Geometry check sheet. Reference: the model listing, model coordinates, mm. A direction names the side the tool comes from. Give positions to 0.01 mm unless a question says otherwise; leave off trailing zeros. Order: outer loops, then holes, each group sorted by start corner. A loop starts at its lowest first (then second) coordinate and runs counter-clockwise, first axis right, second up. Notation, with made-up numbers: M 33.25,7.25 L 51.25,7.25 A21 cw 51.25,41.25 Z; hole C -13.5,89.25 d2. An arc over 180 degrees is marked long. Answer as CSV lines item,"result". Start each with the question number.
Q1. Set-up check for faces 5 (the flat face through (-1, 16, -41)), 6 (the flat face through (-1, 10, -17)), 7 (the flat face through (-1, 29, -41)), 8 (the flat face through (1, 6.9, -41)): record each of +Z, -Z, +X, -X, +Y, -Y from which the full face is reachable in a straight line by a thin tool's end or side.
Q2. Mould release check, pull along Z, two halves, no side actions. Record for faces 1 (the flat face through (-1, 22, -53.532)), 2 (the flat face through (-1, 22, 70.568)), 3 (the flat face through (-3.591, 22, 8)), 4 (the flat face through (-1, 8, -43.793)): +Z half, -Z half, draft (parallel to the pull), parting line (faces both ways), or undercut.
Q3. Section check B-B, the plane z = -14. Record the boundary of the cut face in (x, y).
Q4. Go/stop test with flat-tipped pins: pin 1 (2 mm diameter, centred on x = -0.59, z = -41.19, fed in from -Y); pin 2 (1.4 mm diameter, centred on x = -0.5, z = 58, fed in from +Y). Record where each tip stops, or that it passes through.
Q5. Section check A-A, the plane y = 31.5. Record the boundary of the cut face in (x, z), then the cut area to 3 significant figures.
Q6. Thickness scan on line 1 (Z direction, x = -2.4, y = 4.5); line 2 (Y direction, x = 1.45, z = -43); line 3 (Z direction, x = 0.25, y = 7.5). Record the ranges inside material, lowest first.
Autodesk Inventor part; units mm, degrees
ref_plane "YZ Plane" through (0, 0, 0) normal (1, 0, 0) x (0, 1, 0)
ref_plane "XZ Plane" through (0, 0, 0) normal (0, 1, 0) x (-1, 0, 0)
ref_plane "XY Plane" through (0, 0, 0) normal (0, 0, 1) x (1, 0, 0)
sketch "스케치1" plane through (0, 0, 0) normal (0, 1, 0) x (-1, 0, 0)
  line L0 (3.5912, -53.5318) -> (3.5912, 70.5682)
  line L1 (3.5912, -53.5318) -> (-2.4088, -53.5318)
  line L2 (-2.4088, -53.5318) -> (-2.4088, 70.5682)
  line L3 (-2.4088, 70.5682) -> (3.5912, 70.5682)
  line L4 (3.5912, 70.5682) -> (3.5912, -53.5318)
  point P0 (0, 0)
  dimension "d0" = 6
extrude "돌출1" add sketch "스케치1" along normal blind 45
sketch "스케치2" plane through (0, 45, 0) normal (0, 1, 0) x (1, 0, 0)
  line L0 (2.4088, -70.5682) -> (2.4088, 53.5318)
  line L1 (2.4088, -70.5682) -> (-3.5912, -70.5682)
  line L2 (-3.5912, -70.5682) -> (-3.5912, 53.5318)
  line L3 (-3.5912, 53.5318) -> (2.4088, 53.5318)
  line L4 (2.4088, 53.5318) -> (2.4088, -70.5682)
  circle A0 centre (-0.5912, -58.2682) radius 1.35
  circle A1 centre (-0.5912, 41.1925) radius 1.35
  line L5 (2.4088, -70.5682) -> (2.4088, 53.5318)
  line L6 (2.4088, 53.5318) -> (-3.5912, 53.5318)
  line L7 (-3.5912, 53.5318) -> (-3.5912, -70.5682)
  line L8 (-3.5912, -70.5682) -> (2.4088, -70.5682)
  point P0 (0, 0)
  dimension "d3" = 6
  dimension "d4" = 2.7
  dimension "d5" = 2.7
extrude "돌출2" cut sketch "스케치2" against normal blind 16 contours A0 | A1
sketch "스케치3" plane through (2.4088, 0, 70.5682) normal (1, 0, 0) x (0, 0, -1)
  line L0 (0, 0) -> (124.1, 0)
  line L1 (124.1, 0) -> (124.1, 45)
  line L2 (0, 45) -> (124.1, 45)
  line L3 (0, 0) -> (0, 45)
  line L4 (62.05, 0) -> (77.05, 0)
  line L5 (77.05, 0) -> (47.05, 0)
  line L6 (77.05, 0) -> (97.05, 0)
  line L7 (97.05, 0) -> (97.05, 10)
  line L8 (97.05, 10) -> (77.05, 10)
  line L9 (77.05, 10) -> (77.05, 0)
  line L10 (47.05, 0) -> (27.05, 0)
  line L11 (27.05, 0) -> (27.05, 10)
  line L12 (27.05, 10) -> (47.05, 10)
  line L13 (47.05, 10) -> (47.05, 0)
  point P0 (70.5682, 0)
  dimension "d8" = 15
  dimension "d9" = 30
  dimension "d10" = 20
  dimension "d11" = 10
  dimension "d12" = 20
  dimension "d13" = 10
extrude "돌출3" cut sketch "스케치3" against normal blind 16 contours L11 L12 L13 L0 | L9 L8 L7 L0
sketch "스케치4" plane through (0, 0, 0) normal (0, -1, 0) x (1, 0, 0)
  circle A0 centre (-0.5912, 58.2682) radius 1.35
  circle A1 centre (-0.5912, -41.1925) radius 1.35
  point P0 (0, 0)
extrude "돌출4" cut sketch "스케치4" against normal blind 16
sketch "스케치5" plane through (2.4088, 0, -53.5318) normal (1, 0, 0) x (0, 0, -1)
  line L0 (-97.05, 0) -> (-124.1, 0)
  line L1 (-124.1, 0) -> (-97.05, 0)
  line L2 (-27.05, 0) -> (0, 0)
  line L3 (0, 45) -> (-124.1, 45)
  line L4 (-124.1, 45) -> (0, 45)
  line L5 (-113.15, 45) -> (-110.45, 45)
  line L6 (-13.6892, 45) -> (-10.9892, 45)
  line L7 (-124.1, 45) -> (0, 45)
  line L8 (0, 45) -> (-124.1, 45)
  line L9 (-47.05, 10) -> (-47.05, 0)
  line L10 (-47.05, 0) -> (-77.05, 0)
  line L11 (-77.05, 0) -> (-77.05, 10)
  line L12 (-77.05, 10) -> (-97.05, 10)
  line L13 (-97.05, 10) -> (-97.05, 0)
  line L14 (-97.05, 0) -> (-124.1, 0)
  line L15 (-124.1, 0) -> (-124.1, 45)
  line L16 (0, 45) -> (-124.1, 45)
  line L17 (0, 0) -> (0, 45)
  line L18 (0, 0) -> (-27.05, 0)
  line L19 (-27.05, 0) -> (-27.05, 10)
  line L20 (-27.05, 10) -> (-47.05, 10)
  line L21 (-47.05, 0) -> (-47.05, 10)
  line L22 (-47.05, 10) -> (-27.05, 10)
  line L23 (-27.05, 10) -> (-27.05, 0)
  line L24 (-27.05, 0) -> (0, 0)
  line L25 (0, 0) -> (0, 45)
  line L26 (-124.1, 45) -> (0, 45)
  line L27 (-124.1, 0) -> (-124.1, 45)
  line L28 (-124.1, 0) -> (-97.05, 0)
  line L29 (-97.05, 0) -> (-97.05, 10)
  line L30 (-97.05, 10) -> (-77.05, 10)
  line L31 (-77.05, 10) -> (-77.05, 0)
  line L32 (-77.05, 0) -> (-47.05, 0)
  line L33 (-97.05, 10) -> (-77.05, 10)
  line L34 (-77.05, 10) -> (-97.05, 10)
  line L35 (-77.05, 10) -> (-97.05, 10)
  line L36 (-97.05, 10) -> (-77.05, 10)
  line L37 (-97.05, 10) -> (-97.05, 0)
  line L38 (-97.05, 10) -> (-97.05, 0)
  line L39 (-97.05, 0) -> (-97.05, 10)
  line L40 (-97.05, 0) -> (-97.05, 10)
  line L41 (-110.45, 16) -> (-113.15, 16)
  line L42 (-110.45, 16) -> (-113.15, 16)
  line L43 (-110.45, 0) -> (-113.15, 0)
  line L44 (-110.45, 16) -> (-113.15, 16)
  line L45 (-110.45, 0) -> (-113.15, 0)
  line L46 (-113.15, 29) -> (-110.45, 29)
  line L47 (-113.15, 29) -> (-110.45, 29)
  line L48 (-113.15, 29) -> (-110.45, 29)
  line L49 (-113.15, 45) -> (-110.45, 45)
  line L50 (-110.45, 0) -> (-113.15, 0)
  line L51 (-124.1, 0) -> (-97.05, 0)
  line L52 (-97.05, 0) -> (-124.1, 0)
  line L53 (-124.1, 0) -> (-124.1, 45)
  line L54 (-124.1, 0) -> (-124.1, 45)
  line L55 (-124.1, 0) -> (-124.1, 45)
  line L56 (-124.1, 0) -> (-124.1, 45)
  line L57 (-10.9892, 16) -> (-13.6892, 16)
  line L58 (-10.9892, 16) -> (-13.6892, 16)
  line L59 (-10.9892, 0) -> (-13.6892, 0)
  line L60 (-10.9892, 16) -> (-13.6892, 16)
  line L61 (-10.9892, 0) -> (-13.6892, 0)
  line L62 (0, 0) -> (0, 45)
  line L63 (-10.9892, 0) -> (-13.6892, 0)
  line L64 (0, 0) -> (-27.05, 0)
  line L65 (-27.05, 0) -> (0, 0)
  line L66 (0, 0) -> (-27.05, 0)
  line L67 (-113.15, 45) -> (-110.45, 45)
  line L68 (0, 0) -> (0, 45)
  line L69 (-47.05, 0) -> (-47.05, 10)
  line L70 (-47.05, 10) -> (-47.05, 0)
  line L71 (-47.05, 10) -> (-47.05, 0)
  line L72 (-47.05, 0) -> (-47.05, 10)
  line L73 (-47.05, 10) -> (-27.05, 10)
  line L74 (-27.05, 10) -> (-47.05, 10)
  line L75 (-47.05, 10) -> (-27.05, 10)
  line L76 (-27.05, 0) -> (-27.05, 10)
  line L77 (-27.05, 10) -> (-27.05, 0)
  line L78 (-27.05, 0) -> (-27.05, 10)
  line L79 (-27.05, 10) -> (-27.05, 0)
  line L80 (-13.6892, 45) -> (-10.9892, 45)
  line L81 (-13.6892, 29) -> (-10.9892, 29)
  line L82 (-13.6892, 29) -> (-10.9892, 29)
  line L83 (-13.6892, 45) -> (-10.9892, 45)
  line L84 (0, 0) -> (0, 45)
  line L85 (0, 0) -> (0, 45)
  line L86 (-13.6892, 29) -> (-10.9892, 29)
  line L87 (-77.05, 10) -> (-77.05, 0)
  line L88 (-77.05, 0) -> (-77.05, 10)
  line L89 (-77.05, 10) -> (-77.05, 0)
  line L90 (-77.05, 0) -> (-47.05, 0)
  line L91 (-77.05, 0) -> (-47.05, 0)
  line L92 (-47.05, 0) -> (-77.05, 0)
  line L93 (-47.05, 0) -> (-77.05, 0)
  line L94 (-77.05, 0) -> (-77.05, 10)
  line L95 (-27.05, 10) -> (-47.05, 10)
  line L96 (-13.6892, 0) -> (-13.6892, 16)
  line L97 (-10.9892, 0) -> (-10.9892, 16)
  line L98 (-13.6892, 45) -> (-13.6892, 29)
  line L99 (-10.9892, 45) -> (-10.9892, 29)
  line L100 (-110.45, 45) -> (-110.45, 29)
  line L101 (-113.15, 45) -> (-113.15, 29)
  line L102 (-113.15, 0) -> (-113.15, 16)
  line L103 (-110.45, 0) -> (-110.45, 16)
  line L104 (-9.7392, 6.9) -> (-14.9392, 6.9)
  line L105 (-14.9392, 6.9) -> (-14.9392, 9.1)
  line L106 (-14.9392, 9.1) -> (-9.7392, 9.1)
  line L107 (-9.7392, 9.1) -> (-9.7392, 6.9)
  line L108 (-9.7392, 6.9) -> (-14.9392, 9.1) construction
  line L109 (-14.9392, 6.9) -> (-9.7392, 9.1) construction
  line L110 (-109.2, 9.1) -> (-114.4, 9.1)
  line L111 (-114.4, 9.1) -> (-114.4, 6.9)
  line L112 (-114.4, 6.9) -> (-109.2, 6.9)
  line L113 (-109.2, 6.9) -> (-109.2, 9.1)
  line L114 (-109.2, 9.1) -> (-114.4, 6.9) construction
  line L115 (-114.4, 9.1) -> (-109.2, 6.9) construction
  line L116 (-9.7392, 38.1) -> (-14.9392, 38.1)
  line L117 (-14.9392, 38.1) -> (-14.9392, 35.9)
  line L118 (-14.9392, 35.9) -> (-9.7392, 35.9)
  line L119 (-9.7392, 35.9) -> (-9.7392, 38.1)
  line L120 (-9.7392, 38.1) -> (-14.9392, 35.9) construction
  line L121 (-14.9392, 38.1) -> (-9.7392, 35.9) construction
  line L122 (-109.2, 35.9) -> (-114.4, 35.9)
  line L123 (-114.4, 35.9) -> (-114.4, 38.1)
  line L124 (-114.4, 38.1) -> (-109.2, 38.1)
  line L125 (-109.2, 38.1) -> (-109.2, 35.9)
  line L126 (-109.2, 35.9) -> (-114.4, 38.1) construction
  line L127 (-114.4, 35.9) -> (-109.2, 38.1) construction
  point P0 (-53.5318, 0)
  point P1 (-12.3392, 8)
  point P2 (-111.8, 8)
  point P3 (-12.3392, 37)
  point P4 (-111.8, 37)
  dimension "d18" = 5.2
  dimension "d19" = 2.2
  dimension "d20" = 5.2
  dimension "d21" = 2.2
  dimension "d22" = 5.2
  dimension "d23" = 2.2
extrude "돌출5" cut sketch "스케치5" against normal blind 16 contours L112 L102 L110 L103 | L103 L110 L113 L112 | L112 L111 L110 L102 | L124 L100 L122 L101 | L101 L122 L123 L124 | L124 L125 L122 L100 | L116 L99 L118 L98 | L98 L118 L117 L116 | L116 L119 L118 L99 | L104 L105 L106 L96 | L96 L106 L97 L104 | L97 L106 L107 L104
properties part number "frame_head3" material "PMMA 플라스틱"
Answer block:
1,face 5,"-Y"
1,face 6,"+X, -X, -Y"
1,face 7,"+Y"
1,face 8,"+X, -X"
2,face 1,"-Z half"
2,face 2,"+Z half"
2,face 3,"draft"
2,face 4,"undercut"
3,outline,"M -3.59,10 L 2.41,10 L 2.41,45 L -3.59,45 Z"
4,pin 1,"stops at y = 16"
4,pin 2,"stops at y = 29"
5,outline,"M -3.59,-53.53 L 2.41,-53.53 L 2.41,70.57 L -3.59,70.57 Z; hole C -0.59,-41.19 d2.7; hole C -0.59,58.27 d2.7"
5,area,"733 mm2"
6,line 1,"z = -53.53 to -26.48, -6.48 to 23.52, 43.52 to 70.57"
6,line 2,"y = 0 to 6.9, 9.1 to 35.9, 38.1 to 45"
6,line 3,"z = -53.53 to -43.79, -38.59 to -26.48, -6.48 to 23.52, 43.52 to 55.67, 60.87 to 70.57"
